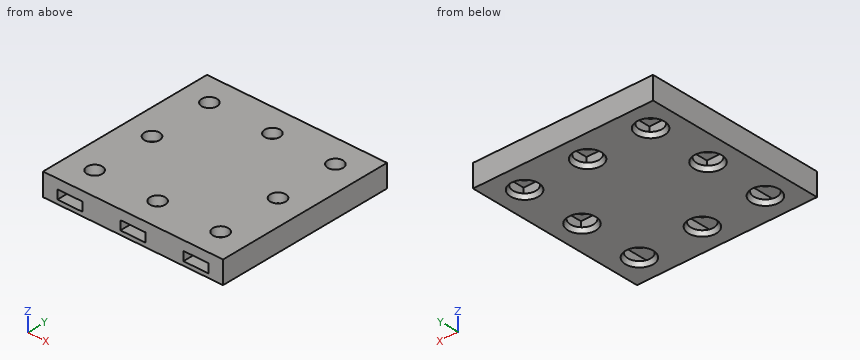
```python
from build123d import *

# Parameters (mm, degrees)
CYLINDER004_R     = 1.7
CYLINDER004_DEPTH = 10
CYLINDER007_R     = 1.7
CYLINDER007_DEPTH = 10
CYLINDER005_R     = 1.7
CYLINDER005_DEPTH = 10
CYLINDER006_R     = 1.7
CYLINDER006_DEPTH = 10
CYLINDER001_R     = 1.7
CYLINDER001_DEPTH = 10
CYLINDER002_R     = 1.7
CYLINDER002_DEPTH = 10
CYLINDER003_R     = 1.7
CYLINDER003_DEPTH = 10
CYLINDER_R        = 1.7
CYLINDER_DEPTH    = 10
BOX065_W          = 5.8
BOX065_H          = 5.8
BOX065_DEPTH      = 2
BOX062_W          = 5.4
BOX062_H          = 5.4
BOX062_DEPTH      = 2
BOX063_W          = 5.7
BOX063_H          = 5.7
BOX063_DEPTH      = 2
BOX064_W          = 5.5
BOX064_H          = 5.5
BOX064_DEPTH      = 2
BOX066_W          = 5.6
BOX066_H          = 10
BOX066_DEPTH      = 2
BOX059_W          = 5.6
BOX059_H          = 5.6
BOX059_DEPTH      = 2
BOX060_W          = 5.6
BOX060_H          = 10
BOX060_DEPTH      = 2
BOX061_W          = 5.6
BOX061_H          = 10
BOX061_DEPTH      = 2
BOX058_W          = 40
BOX058_H          = 40
BOX058_DEPTH      = 5


with BuildPart() as cylinder004:
    # Cylinder004 → Cylinder004 (new body)
    with BuildSketch(Plane(origin=(20, 34, 0), x_dir=(1, 0, 0), z_dir=(0, 0, 1))):
        Circle(CYLINDER004_R)
    extrude(amount=CYLINDER004_DEPTH)


with BuildPart() as cylinder007:
    # Cylinder007 → Cylinder007 (new body)
    with BuildSketch(Plane(origin=(34, 20, 0), x_dir=(1, 0, 0), z_dir=(0, 0, 1))):
        Circle(CYLINDER007_R)
    extrude(amount=CYLINDER007_DEPTH)


with BuildPart() as cylinder005:
    # Cylinder005 → Cylinder005 (new body)
    with BuildSketch(Plane(origin=(6, 34, 0), x_dir=(1, 0, 0), z_dir=(0, 0, 1))):
        Circle(CYLINDER005_R)
    extrude(amount=CYLINDER005_DEPTH)


with BuildPart() as cylinder006:
    # Cylinder006 → Cylinder006 (new body)
    with BuildSketch(Plane(origin=(6, 20, 0), x_dir=(1, 0, 0), z_dir=(0, 0, 1))):
        Circle(CYLINDER006_R)
    extrude(amount=CYLINDER006_DEPTH)


with BuildPart() as cylinder001:
    # Cylinder001 → Cylinder001 (new body)
    with BuildSketch(Plane(origin=(20, 6, 0), x_dir=(1, 0, 0), z_dir=(0, 0, 1))):
        Circle(CYLINDER001_R)
    extrude(amount=CYLINDER001_DEPTH)


with BuildPart() as cylinder002:
    # Cylinder002 → Cylinder002 (new body)
    with BuildSketch(Plane(origin=(34, 6, 0), x_dir=(1, 0, 0), z_dir=(0, 0, 1))):
        Circle(CYLINDER002_R)
    extrude(amount=CYLINDER002_DEPTH)


with BuildPart() as cylinder003:
    # Cylinder003 → Cylinder003 (new body)
    with BuildSketch(Plane(origin=(34, 34, 0), x_dir=(1, 0, 0), z_dir=(0, 0, 1))):
        Circle(CYLINDER003_R)
    extrude(amount=CYLINDER003_DEPTH)


with BuildPart() as fusion018:
    # Cylinder → Cylinder (new body)
    with BuildSketch(Plane(origin=(6, 6, 0), x_dir=(1, 0, 0), z_dir=(0, 0, 1))):
        Circle(CYLINDER_R)
    extrude(amount=CYLINDER_DEPTH)

    # Fusion018: union Cylinder004, Cylinder007, Cylinder005, Cylinder006, Cylinder001, Cylinder002, Cylinder003
    add(cylinder004.part)
    add(cylinder007.part)
    add(cylinder005.part)
    add(cylinder006.part)
    add(cylinder001.part)
    add(cylinder002.part)
    add(cylinder003.part)


with BuildPart() as sphere024:
    # Sphere024 → Sphere024 (revolve)
    with BuildSketch(Plane(origin=(6, 34, 2.4), x_dir=(1, 0, 0), z_dir=(0, -1, 0))):
        with BuildLine():
            ThreePointArc((0, -3.35), (3.35, 0), (0, 3.35))
            Line((0, 3.35), (0, -3.35))
        make_face()
    revolve(axis=Axis((6, 34, 2.4), (0, 0, 1)))


with BuildPart() as obj1:
    # Sphere006 → Sphere006 (revolve)
    with BuildSketch(Plane(origin=(6, 6, 2.4), x_dir=(1, 0, 0), z_dir=(0, -1, 0))):
        with BuildLine():
            ThreePointArc((0, -3.35), (3.35, 0), (0, 3.35))
            Line((0, 3.35), (0, -3.35))
        make_face()
    revolve(axis=Axis((6, 6, 2.4), (0, 0, 1)))


with BuildPart() as sphere025:
    # Sphere025 → Sphere025 (revolve)
    with BuildSketch(Plane(origin=(20, 6, 2.4), x_dir=(1, 0, 0), z_dir=(0, -1, 0))):
        with BuildLine():
            ThreePointArc((0, -3.35), (3.35, 0), (0, 3.35))
            Line((0, 3.35), (0, -3.35))
        make_face()
    revolve(axis=Axis((20, 6, 2.4), (0, 0, 1)))


with BuildPart() as sphere001:
    # Sphere001 → Sphere001 (revolve)
    with BuildSketch(Plane(origin=(34, 6, 2.4), x_dir=(1, 0, 0), z_dir=(0, -1, 0))):
        with BuildLine():
            ThreePointArc((0, -3.35), (3.35, 0), (0, 3.35))
            Line((0, 3.35), (0, -3.35))
        make_face()
    revolve(axis=Axis((34, 6, 2.4), (0, 0, 1)))


with BuildPart() as sphere026:
    # Sphere026 → Sphere026 (revolve)
    with BuildSketch(Plane(origin=(20, 34, 2.4), x_dir=(1, 0, 0), z_dir=(0, -1, 0))):
        with BuildLine():
            ThreePointArc((0, -3.35), (3.35, 0), (0, 3.35))
            Line((0, 3.35), (0, -3.35))
        make_face()
    revolve(axis=Axis((20, 34, 2.4), (0, 0, 1)))


with BuildPart() as sphere004:
    # Sphere004 → Sphere004 (revolve)
    with BuildSketch(Plane(origin=(6, 20, 2.4), x_dir=(1, 0, 0), z_dir=(0, -1, 0))):
        with BuildLine():
            ThreePointArc((0, -3.35), (3.35, 0), (0, 3.35))
            Line((0, 3.35), (0, -3.35))
        make_face()
    revolve(axis=Axis((6, 20, 2.4), (0, 0, 1)))


with BuildPart() as sphere002:
    # Sphere002 → Sphere002 (revolve)
    with BuildSketch(Plane(origin=(34, 34, 2.4), x_dir=(1, 0, 0), z_dir=(0, -1, 0))):
        with BuildLine():
            ThreePointArc((0, -3.35), (3.35, 0), (0, 3.35))
            Line((0, 3.35), (0, -3.35))
        make_face()
    revolve(axis=Axis((34, 34, 2.4), (0, 0, 1)))


with BuildPart() as fusion019:
    # Sphere007 → Sphere007 (revolve)
    with BuildSketch(Plane(origin=(34, 20, 2.4), x_dir=(1, 0, 0), z_dir=(0, -1, 0))):
        with BuildLine():
            ThreePointArc((0, -3.35), (3.35, 0), (0, 3.35))
            Line((0, 3.35), (0, -3.35))
        make_face()
    revolve(axis=Axis((34, 20, 2.4), (0, 0, 1)))

    # Fusion019: union Sphere024, obj1, Sphere025, Sphere001, Sphere026, Sphere004, Sphere002
    add(sphere024.part)
    add(obj1.part)
    add(sphere025.part)
    add(sphere001.part)
    add(sphere026.part)
    add(sphere004.part)
    add(sphere002.part)


with BuildPart() as box065:
    # Box065 → Box065 (new body)
    with BuildSketch(Plane(origin=(3.1, 17.1, 4.6), x_dir=(1, 0, 0), z_dir=(0, 0, 1))):
        with Locations((2.9, 2.9)):
            Rectangle(BOX065_W, BOX065_H)
    extrude(amount=BOX065_DEPTH)


with BuildPart() as box062:
    # Box062 → Box062 (new body)
    with BuildSketch(Plane(origin=(31.3, 17.3, 4.6), x_dir=(1, 0, 0), z_dir=(0, 0, 1))):
        with Locations((2.7, 2.7)):
            Rectangle(BOX062_W, BOX062_H)
    extrude(amount=BOX062_DEPTH)


with BuildPart() as box063:
    # Box063 → Box063 (new body)
    with BuildSketch(Plane(origin=(3.15, 31.15, 4.6), x_dir=(1, 0, 0), z_dir=(0, 0, 1))):
        with Locations((2.85, 2.85)):
            Rectangle(BOX063_W, BOX063_H)
    extrude(amount=BOX063_DEPTH)


with BuildPart() as box064:
    # Box064 → Box064 (new body)
    with BuildSketch(Plane(origin=(31.25, 31.25, 4.6), x_dir=(1, 0, 0), z_dir=(0, 0, 1))):
        with Locations((2.75, 2.75)):
            Rectangle(BOX064_W, BOX064_H)
    extrude(amount=BOX064_DEPTH)


with BuildPart() as box066:
    # Box066 → Box066 (new body)
    with BuildSketch(Plane(origin=(3.2, -0.85, 4.6), x_dir=(1, 0, 0), z_dir=(0, 0, 1))):
        with Locations((2.8, 5)):
            Rectangle(BOX066_W, BOX066_H)
    extrude(amount=BOX066_DEPTH)


with BuildPart() as box059:
    # Box059 → Box059 (new body)
    with BuildSketch(Plane(origin=(17.2, 31.2, 4.6), x_dir=(1, 0, 0), z_dir=(0, 0, 1))):
        with Locations((2.8, 2.8)):
            Rectangle(BOX059_W, BOX059_H)
    extrude(amount=BOX059_DEPTH)


with BuildPart() as box060:
    # Box060 → Box060 (new body)
    with BuildSketch(Plane(origin=(17.2, -0.85, 4.6), x_dir=(1, 0, 0), z_dir=(0, 0, 1))):
        with Locations((2.8, 5)):
            Rectangle(BOX060_W, BOX060_H)
    extrude(amount=BOX060_DEPTH)


with BuildPart() as fusion020:
    # Box061 → Box061 (new body)
    with BuildSketch(Plane(origin=(31.2, -0.85, 4.6), x_dir=(1, 0, 0), z_dir=(0, 0, 1))):
        with Locations((2.8, 5)):
            Rectangle(BOX061_W, BOX061_H)
    extrude(amount=BOX061_DEPTH)

    # Fusion020: union Box065, Box062, Box063, Box064, Box066, Box059, Box060
    add(box065.part)
    add(box062.part)
    add(box063.part)
    add(box064.part)
    add(box066.part)
    add(box059.part)
    add(box060.part)


with BuildPart() as cut018:
    # Box058 → Box058 (new body)
    with BuildSketch(Plane.XY.offset(3.7)):
        with Locations((20, 20)):
            Rectangle(BOX058_W, BOX058_H)
    extrude(amount=BOX058_DEPTH)

    # Cut017: cut Fusion020
    add(fusion020.part, mode=Mode.SUBTRACT)

    # Cut019: cut Fusion019
    add(fusion019.part, mode=Mode.SUBTRACT)

    # Cut018: cut Fusion018
    add(fusion018.part, mode=Mode.SUBTRACT)


solid = cut018.part
```
Could you check a few things on this model? Use its own coordinates, in mm. Give positions to 0.01 mm unless a question says otherwise; leave off trailing zeros. Order: outer loops, then holes, each group sorted by start corner. A loop starts at its lowest first (then second) coordinate and runs counter-clockwise, first axis right, second up.
Q1. Suppose I cut it at B-B, the plane z = 5.7. Count the separate pieces of the cut face and the enclosed holes in it, and give its area (3 significant figures).
Q2. Suppose I cut it at A-A, the plane y = 20. Write out the boundary of the cut face in (x, z), and give its area (3 significant figures).
Q3. If I drill on line 1 along X through (y, z) = (31.5, 6.55); line 2 along Y through (x, z) = (34, 8.1); line 3 along Y through (x, z) = (5, 5.9), over which ranges is the centre line in solid material (lowest first)?
Q4. I'm going to push flat-ended pins straight in: P1, Ø6, axis at x = 5, y = 6, coming from the -Z side; P2, Ø1.6, axis at x = 34.5, y = 21, coming from the -Z side; P3, Ø1, axis at x = 19.5, z = 6, coming from the -Y side. Where does each tip first touch, or does it pass through?
Solution:
1. separate pieces: 1
1. enclosed holes: 5
1. area: 1,290 mm2
2. outline: (0, 3.7) - (2.91, 3.7) arc R3.35 cw to (3.47, 4.6) - (3.1, 4.6) - (3.1, 6.6) - (4.3, 6.6) - (4.3, 8.7) - (0, 8.7) - close; (7.7, 6.6) - (8.9, 6.6) - (8.9, 4.6) - (8.53, 4.6) arc R3.35 cw to (9.09, 3.7) - (30.91, 3.7) arc R3.35 cw to (31.47, 4.6) - (31.3, 4.6) - (31.3, 6.6) - (32.3, 6.6) - (32.3, 8.7) - (7.7, 8.7) - close; (35.7, 6.6) - (36.7, 6.6) - (36.7, 4.6) - (36.53, 4.6) arc R3.35 cw to (37.09, 3.7) - (40, 3.7) - (40, 8.7) - (35.7, 8.7) - close
2. area: 153 mm2
3. line 1: x = 0 to 3.15, 8.85 to 17.2, 22.8 to 31.25, 36.75 to 40
3. line 2: y = 0 to 4.3, 7.7 to 18.3, 21.7 to 32.3, 35.7 to 40
3. line 3: y = 9.15 to 17.1, 22.9 to 31.15, 36.85 to 40
4. P1: stops at z = 3.7
4. P2: stops at z = 6.6
4. P3: stops at y = 9.15
